Can you work these out from the model? Positions are in its coordinate system, mm. Face numbers are marked on the shaded views. A direction names the side the tool comes from. Coordinates: 2 decimals unless noted, no trailing zeros. Write each loop counter-clockwise with the first axis right and the second up, starting at its lowest first coordinate (ties: lowest second). Pieces come first, ordered by that corner, then holes. Notation, with made-up numbers: (87, 40) - (138, 40) arc R14 ccw to (138, 44) - close; hole circle Ø9 at (-29.5, -12.75). An arc over 180 degrees is marked (long way). Use one line per item in the form item = value. Start each with the question number.
(1) Thinking about a two-plate mould opening in X: for the marked faces 1, 2, 3 and 4, which applies, pulls with the +X half, pulls with the -X half, needs draft (parallel to the pull), parting line crosses it, or undercut?
(2) If I drill on probe 1 along X at (y, z) = (42, 13); probe 2 along X at (y, z) = (46, -17.5); probe 3 along Y at (x, z) = (-69, 8), over which ranges is the centre line in solid material (lowest first)? Write a range as from..to.
(3) For pin 1 Ø1 at (x, z) = (-25, 6) entering from -Y; pin 2 Ø21.5 at (x, y) = (1, 21.5) entering from +Z; pin 3 Ø21.5 at (y, z) = (27, -7.5) entering from +X, each with a flat end and sliding along its axis, tell me the tip position at first contact or that it passes through.
(4) If we section it at D-D on x = -7.5: Please give me the cut outline in (y, z), then the cut area to 4 significant figures.
(5) If we section it at B-B on y = 41: Please give me the cut outline in (x, z), then the cut area to 3 significant figures.
(6) On a 3-axis mill with a long thin cutter (end or side, diameter ignored), from which of +Z, -Z, +X, -X, +Y, -Y can I reach the whole of each face in a straight line? I mean the marked faces 5 and 6. Say none if no direction works.
(7) If we section it at C-C on y = 24.5: Please give me the cut outline in (x, z), then the cut area to 3 significant figures.
(8) If we section it at A-A on z = -6.5: Please give me the cut outline in (x, y), then the cut area to 3 significant figures.
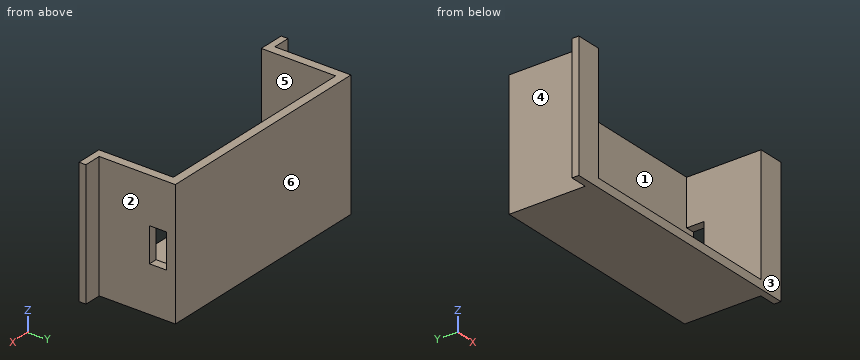
```python
from build123d import *

# Parameters (mm, degrees)
SKETCH_1_W          = 132.5
SKETCH_1_H          = 73.1
EXTRUDE_1_DEPTH     = 48.2
SKETCH_3_W          = 122.5
SKETCH_3_H          = 43.2
CUT_EXTRUDE_1_DEPTH = 68.1
SKETCH_7_W          = 20
SKETCH_7_H          = 10
CUT_EXTRUDE_2_DEPTH = 10
SKETCH_8_W          = 73.1
SKETCH_8_H          = 4
EXTRUDE_2_DEPTH     = 10
SKETCH_9_W          = 73.1
SKETCH_9_H          = 4
EXTRUDE_3_DEPTH     = 10


with BuildPart() as part:
    # 草圖1 → 填料-伸長1 (new body)
    with BuildSketch(Plane(origin=(0, 0, 0), x_dir=(1, 0, 0), z_dir=(0, 1, 0))):
        Rectangle(SKETCH_1_W, SKETCH_1_H)
    extrude(amount=EXTRUDE_1_DEPTH)

    # 草圖3 → 除料-伸長1 (cut)
    with BuildSketch(Plane.XY.offset(36.55)):
        with Locations((0, 21.6)):
            Rectangle(SKETCH_3_W, SKETCH_3_H)
    extrude(amount=-CUT_EXTRUDE_1_DEPTH, mode=Mode.SUBTRACT)

    # 草圖7 → 除料-伸長2 (cut)
    with BuildSketch(Plane(origin=(66.25, 0, 0), x_dir=(0, 0, -1), z_dir=(1, 0, 0))):
        with Locations((0, 38.2)):
            Rectangle(SKETCH_7_W, SKETCH_7_H)
    extrude(amount=-CUT_EXTRUDE_2_DEPTH, mode=Mode.SUBTRACT)

    # 草圖8 → 填料-伸長2 (add)
    with BuildSketch(Plane(origin=(66.25, 0, 0), x_dir=(0, 0, -1), z_dir=(1, 0, 0))):
        with Locations((0, 2)):
            Rectangle(SKETCH_8_W, SKETCH_8_H)
    extrude(amount=EXTRUDE_2_DEPTH)

    # 草圖9 → 填料-伸長3 (add)
    with BuildSketch(Plane.ZY.offset(66.25)):
        with Locations((0, 2)):
            Rectangle(SKETCH_9_W, SKETCH_9_H)
    extrude(amount=EXTRUDE_3_DEPTH)


solid = part.part
```
Reported:
q1.face_1 = undercut
q1.face_2 = pulls with the +X half
q1.face_3 = needs draft
q1.face_4 = pulls with the -X half
q2.probe_1 = -66.25..-61.25, 61.25..66.25
q2.probe_2 = -66.25..66.25
q2.probe_3 = 0..4
q3.pin_1 = 43.2
q3.pin_2 = -31.55
q3.pin_3 = 66.25
q4.outline = (0, -36.55) - (48.2, -36.55) - (48.2, 36.55) - (43.2, 36.55) - (43.2, -31.55) - (0, -31.55) - close
q4.area = 581.5 mm2
q5.outline = (-66.25, -36.55) - (66.25, -36.55) - (66.25, -10) - (61.25, -10) - (61.25, -31.55) - (-61.25, -31.55) - (-61.25, 36.55) - (-66.25, 36.55) - close; (61.25, 10) - (66.25, 10) - (66.25, 36.55) - (61.25, 36.55) - close
q5.area = 1,240 mm2
q6.face_5 = +Z, -Y
q6.face_6 = +Z, -Z, +X, -X, +Y
q7.outline = (-66.25, -36.55) - (66.25, -36.55) - (66.25, 36.55) - (61.25, 36.55) - (61.25, -31.55) - (-61.25, -31.55) - (-61.25, 36.55) - (-66.25, 36.55) - close
q7.area = 1,340 mm2
q8.outline = (-76.25, 0) - (-61.25, 0) - (-61.25, 43.2) - (66.25, 43.2) - (66.25, 48.2) - (-66.25, 48.2) - (-66.25, 4) - (-76.25, 4) - close; (61.25, 0) - (76.25, 0) - (76.25, 4) - (66.25, 4) - (66.25, 33.2) - (61.25, 33.2) - close
q8.area = 1,120 mm2
